Study the drawing (mm; zero at the part's minimum x, y, z) and answer. Coordinates: 2 decimals unless noted, no trailing zeros. Loops run counter-clockwise (first coordinate to the right, second up) from the corner with the lowest first, then second, coordinate; pieces in that order, holes last. Notation, with made-up numbers: (14.25, 31) - (41.25, 31) arc R17 cw to (41.25, 54) - close; hole circle Ø1 at (79.25, -17.5). An arc over 180 degrees is marked (long way). Put each result on its own line as item: value.
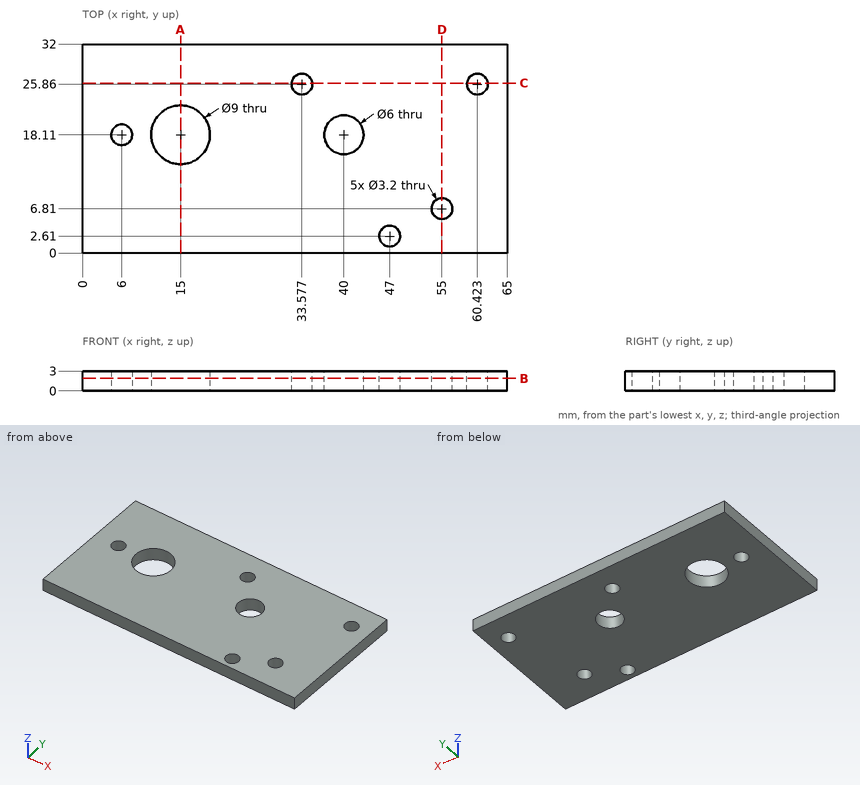
1) The part is cut by section A-A (x = 15). Give the vertices of the cut face in (y, z), and give its area (3 significant figures).
Found:
outline: (0, 0) - (13.61, 0) - (13.61, 3) - (0, 3) - close; (22.61, 0) - (32, 0) - (32, 3) - (22.61, 3) - close
area: 69.0 mm^2
2) Straight lines are drawn through the part: L1, parallel to X at y = 18, z = 0.9; L2, parallel to Y at x = 6, z = 2.15; L3, parallel to Y at x = 33.5, z = 2. For each, find the intervals that lie inside material, in ascending order. Write a range as [from, to].
Found:
L1: x = [0, 4.4], [7.6, 10.5], [19.5, 37], [43, 65]
L2: y = [0, 16.51], [19.71, 32]
L3: y = [0, 24.26], [27.46, 32]
3) The part is cut by section B-B (z = 1.9). Give the vertices of the cut face in (x, y).
Found:
outline: (0, 0) - (65, 0) - (65, 32) - (0, 32) - close; hole circle Ø3.2 at (6, 18.11); hole circle Ø9 at (15, 18.11); hole circle Ø3.2 at (33.58, 25.86); hole circle Ø6 at (40, 18.11); hole circle Ø3.2 at (47, 2.61); hole circle Ø3.2 at (55, 6.81); hole circle Ø3.2 at (60.42, 25.86)
4) The part is cut by section D-D (x = 55). Give the vertices of the cut face in (y, z).
Found:
outline: (0, 0) - (5.21, 0) - (5.21, 3) - (0, 3) - close; (8.41, 0) - (32, 0) - (32, 3) - (8.41, 3) - close
5) The part is cut by section C-C (y = 26). Give the vertices of the cut face in (x, z), and give its area (3 significant figures).
Found:
outline: (0, 0) - (31.98, 0) - (31.98, 3) - (0, 3) - close; (35.17, 0) - (58.83, 0) - (58.83, 3) - (35.17, 3) - close; (62.02, 0) - (65, 0) - (65, 3) - (62.02, 3) - close
area: 176 mm^2
